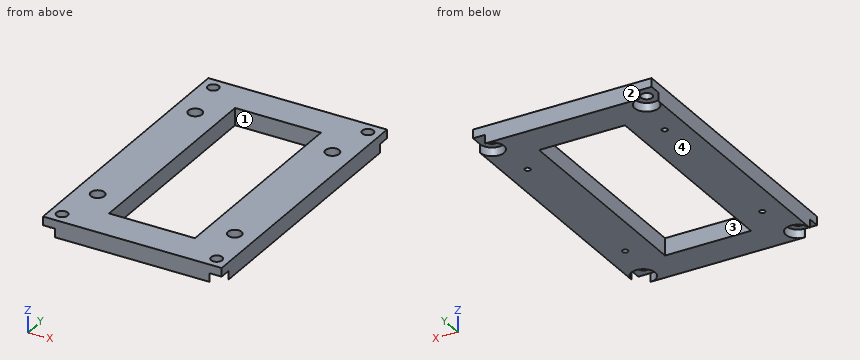
```python
from build123d import *

# Parameters (mm, degrees)
SKETCH1_W           = 104
SKETCH1_H           = 164
SKETCH1_R           = 3.25
BOSS_EXTRUDE1_DEPTH = 10
SKETCH2_R           = 1.625
CUT_EXTRUDE1_DEPTH  = 10
SKETCH3_R           = 4
CUT_EXTRUDE2_DEPTH  = 5
SKETCH5_R           = 7
SKETCH5_R_2         = 3.25
CUT_EXTRUDE3_DEPTH  = 5
SKETCH6_W           = 50
SKETCH6_H           = 125
CUT_EXTRUDE4_DEPTH  = 52


with BuildPart() as part:
    # Sketch1 → Boss-Extrude1 (new body)
    with BuildSketch(Plane.XY):
        Rectangle(SKETCH1_W, SKETCH1_H)
        with Locations((-45, 75)):
            Circle(SKETCH1_R, mode=Mode.SUBTRACT)
        with Locations((45, 75)):
            Circle(SKETCH1_R, mode=Mode.SUBTRACT)
        with Locations((-45, -75)):
            Circle(SKETCH1_R, mode=Mode.SUBTRACT)
        with Locations((45, -75)):
            Circle(SKETCH1_R, mode=Mode.SUBTRACT)
    extrude(amount=BOSS_EXTRUDE1_DEPTH)

    # Sketch2 → Cut-Extrude1 (cut)
    with BuildSketch(Plane(origin=(0, 0, 0), x_dir=(-1, 0, 0), z_dir=(0, 0, -1))):
        with Locations((-39.9, 48.4)):
            Circle(SKETCH2_R)
        with Locations((39.9, 48.4)):
            Circle(SKETCH2_R)
        with Locations((-39.9, -48.4)):
            Circle(SKETCH2_R)
        with Locations((39.9, -48.4)):
            Circle(SKETCH2_R)
    extrude(amount=-CUT_EXTRUDE1_DEPTH, mode=Mode.SUBTRACT)

    # Sketch3 → Cut-Extrude2 (cut)
    with BuildSketch(Plane.XY.offset(10)):
        with Locations((-39.9, 48.4)):
            Circle(SKETCH3_R)
        with Locations((39.9, 48.4)):
            Circle(SKETCH3_R)
        with Locations((-39.9, -48.4)):
            Circle(SKETCH3_R)
        with Locations((39.9, -48.4)):
            Circle(SKETCH3_R)
    extrude(amount=-CUT_EXTRUDE2_DEPTH, mode=Mode.SUBTRACT)

    # Sketch5 → Cut-Extrude3 (cut)
    # profile 1 of 8: a face of its own
    with BuildSketch(Plane(origin=(0, 0, 0), x_dir=(-1, 0, 0), z_dir=(0, 0, -1))):
        with Locations((-45, 75)):
            Circle(SKETCH5_R)
        with Locations((-45, 75)):
            Circle(SKETCH5_R_2, mode=Mode.SUBTRACT)
    # profile 2 of 8: a face of its own
    with BuildSketch(Plane(origin=(0, 0, 0), x_dir=(-1, 0, 0), z_dir=(0, 0, -1))):
        with BuildLine():
            Line((-44.999999978, 82), (-52, 82))
            Line((-52, 82), (-52, 75))
            ThreePointArc((-52, 75), (-49.94974746, 79.949747476), (-44.999999978, 82))
        make_face()
    # profile 3 of 8: a face of its own
    with BuildSketch(Plane(origin=(0, 0, 0), x_dir=(-1, 0, 0), z_dir=(0, 0, -1))):
        with Locations((45, 75)):
            Circle(SKETCH5_R)
        with Locations((45, 75)):
            Circle(SKETCH5_R_2, mode=Mode.SUBTRACT)
    # profile 4 of 8: a face of its own
    with BuildSketch(Plane(origin=(0, 0, 0), x_dir=(-1, 0, 0), z_dir=(0, 0, -1))):
        with BuildLine():
            Line((52, 82), (45, 82))
            ThreePointArc((45, 82), (49.949747468, 79.949747468), (52, 75))
            Line((52, 75), (52, 82))
        make_face()
    # profile 5 of 8: a face of its own
    with BuildSketch(Plane(origin=(0, 0, 0), x_dir=(-1, 0, 0), z_dir=(0, 0, -1))):
        with Locations((-45, -75)):
            Circle(SKETCH5_R)
        with Locations((-45, -75)):
            Circle(SKETCH5_R_2, mode=Mode.SUBTRACT)
    # profile 6 of 8: a face of its own
    with BuildSketch(Plane(origin=(0, 0, 0), x_dir=(-1, 0, 0), z_dir=(0, 0, -1))):
        with Locations((45, -75)):
            Circle(SKETCH5_R)
        with Locations((45, -75)):
            Circle(SKETCH5_R_2, mode=Mode.SUBTRACT)
    # profile 7 of 8: a face of its own
    with BuildSketch(Plane(origin=(0, 0, 0), x_dir=(-1, 0, 0), z_dir=(0, 0, -1))):
        with BuildLine():
            Line((52, -82), (52, -75))
            ThreePointArc((52, -75), (49.949747468, -79.949747468), (45, -82))
            Line((45, -82), (52, -82))
        make_face()
    # profile 8 of 8: a face of its own
    with BuildSketch(Plane(origin=(0, 0, 0), x_dir=(-1, 0, 0), z_dir=(0, 0, -1))):
        with BuildLine():
            ThreePointArc((-45, -82), (-49.949747468, -79.949747468), (-52, -75))
            Line((-52, -75), (-52, -82))
            Line((-52, -82), (-45, -82))
        make_face()
    extrude(amount=-CUT_EXTRUDE3_DEPTH, mode=Mode.SUBTRACT)

    # Sketch6 → Cut-Extrude4 (cut)
    with BuildSketch(Plane(origin=(0, 0, 0), x_dir=(-1, 0, 0), z_dir=(0, 0, -1))):
        Rectangle(SKETCH6_W, SKETCH6_H)
    extrude(amount=-CUT_EXTRUDE4_DEPTH, mode=Mode.SUBTRACT)


solid = part.part
```
Input: part model. Units: mm. Frame: model coordinates. Face numbers are marked on the shaded views. Round coordinates to 2 decimals unless told otherwise and drop trailing zeros. Order: outer loops, then holes, each group sorted by start corner. A loop starts at its lowest first (then second) coordinate and runs counter-clockwise, first axis right, second up. Notation, with made-up numbers: (54.5, 8.5) - (102.5, 8.5) arc R13 cw to (102.5, 20.5) - close; hole circle Ø11 at (40, 71.25). An arc over 180 degrees is marked (long way). One line per question, with ' | ' between items. Start each with the question number.
1) Contact query for flat-ended pins moving along their axis: P1, Ø2.5, axis at x = 41, y = 47, coming from the +Z side; P2, Ø4, axis at x = -45.5, y = 78, coming from the -Z side. Output: stop coordinate, or through.
2) Cut plane A-A, the plane y = -14. Return the cut outline in (x, z), then the cut area to 3 significant figures.
3) Cut plane C-C, the plane x = -18.5. Return the cut outline in (y, z), then the cut area to 3 significant figures.
4) Ray query, probe 1 along Y at (x, z) = (-39.9, 6.9); probe 2 along Y at (x, z) = (-45, 8.75); probe 3 along Y at (x, z) = (10.5, 1). Return the intervals inside material, ascending.
5) Cut plane B-B, the plane y = 48.4. Return the cut outline in (x, z) (3 decimals), then the cut area to 4 significant figures.
6) Pull-direction query (Y, two-part tool) for the marked faces 1, 2, 3 and 4; classes: +Y half, -Y half, draft (parallel to the pull), parting line (faces both ways), or undercut.
7) Cut plane D-D, the plane x = 39.9. Return the cut outline in (y, z) (3 decimals).
Worked out:
1) P1: stops at z = 5 | P2: stops at z = 5
2) outline: (-52, 0) - (-25, 0) - (-25, 10) - (-52, 10) - close; (25, 0) - (52, 0) - (52, 10) - (25, 10) - close | area: 540 mm^2
3) outline: (-82, 0) - (-62.5, 0) - (-62.5, 10) - (-82, 10) - close; (62.5, 0) - (82, 0) - (82, 10) - (62.5, 10) - close | area: 390 mm^2
4) probe 1: y = -82 to -52.4, -44.4 to 44.4, 52.4 to 82 | probe 2: y = -82 to -78.25, -71.75 to 71.75, 78.25 to 82 | probe 3: y = -82 to -62.5, 62.5 to 82
5) outline: (-52, 0) - (-41.525, 0) - (-41.525, 5) - (-43.9, 5) - (-43.9, 10) - (-52, 10) - close; (-38.275, 0) - (-25, 0) - (-25, 10) - (-35.9, 10) - (-35.9, 5) - (-38.275, 5) - close; (25, 0) - (38.275, 0) - (38.275, 5) - (35.9, 5) - (35.9, 10) - (25, 10) - close; (41.525, 0) - (52, 0) - (52, 10) - (43.9, 10) - (43.9, 5) - (41.525, 5) - close | area: 427.5 mm^2
6) face 1: undercut | face 2: +Y half | face 3: undercut | face 4: draft
7) outline: (-82, 0) - (-79.795, 0) - (-79.795, 5) - (-70.205, 5) - (-70.205, 0) - (-50.025, 0) - (-50.025, 5) - (-52.4, 5) - (-52.4, 10) - (-82, 10) - close; (-46.775, 0) - (46.775, 0) - (46.775, 5) - (44.4, 5) - (44.4, 10) - (-44.4, 10) - (-44.4, 5) - (-46.775, 5) - close; (50.025, 0) - (70.205, 0) - (70.205, 5) - (79.795, 5) - (79.795, 0) - (82, 0) - (82, 10) - (52.4, 10) - (52.4, 5) - (50.025, 5) - close
